Design review of the part shown in the three views and the two pictorial views. Dimensions are in mm from the part's minimum x, y and z. A direction names the side the tool comes from. Coordinates: 2 decimals unless noted, no trailing zeros. Write each loop counter-clockwise with the first axis right and the second up, starting at its lowest first coordinate (ties: lowest second). Pieces come first, ordered by that corner, then holes. Notation, with made-up numbers: (66.25, -32.5) -> (71.25, -32.5) arc R8 ccw to (71.25, -19.5) -> close; hole circle Ø11 at (13.5, 76). An arc over 180 degrees is marked (long way). Write each question's results on one line, items separated by ' | '.
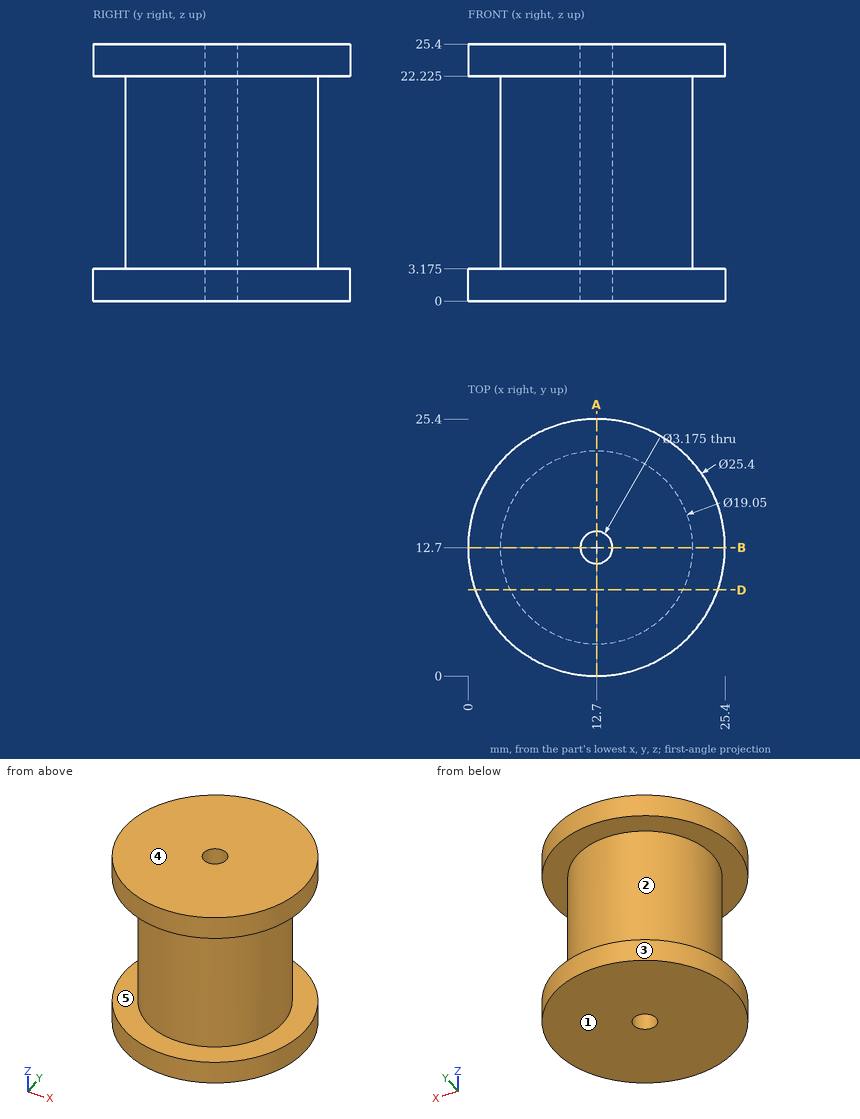
Q1. Add section D-D (y = 8.5). Write out the cut boundary in (x, z) (3 decimals), plus the area to 3 significant figures.
Solution:
outline: (0.715, 0) -> (24.685, 0) -> (24.685, 3.175) -> (21.249, 3.175) -> (21.249, 22.225) -> (24.685, 22.225) -> (24.685, 25.4) -> (0.715, 25.4) -> (0.715, 22.225) -> (4.151, 22.225) -> (4.151, 3.175) -> (0.715, 3.175) -> close | area: 478 mm²
Q2. For line 1 (Y direction, x = 12.7, z = 9.25) (1 decimal); line 2 (Y direction, x = 12.25, z = 23.5); line 3 (Z direction, x = 6.5, y = 23) (3 decimals), list the stretches that pass through material, from the lowest coordinate up. Write a range as from..to.
Solution:
line 1: 3.2..11.1, 14.3..22.2 | line 2: 0.01..11.18, 14.22..25.39 | line 3: 0..3.175, 22.225..25.4
Q3. Clearance check with flat-ended pins moving along their axes: P1, Ø1, axis at x = 15, z = 22.5, coming from the -Y side; P2, Ø4, axis at y = 5.5, z = 6, coming from the -X side; P3, Ø1.5, axis at y = 5, z = 2.5, coming from the -X side. State where each tip first meets the part, or that it passes through.
Solution:
P1: y = 0.13 | P2: x = 4.72 | P3: x = 2.07
Q4. Add section A-A (x = 12.7). Write out the cut boundary in (y, z) (1 decimal).
Solution:
outline: (0, 0) -> (11.1, 0) -> (11.1, 25.4) -> (0, 25.4) -> (0, 22.2) -> (3.2, 22.2) -> (3.2, 3.2) -> (0, 3.2) -> close; (14.3, 0) -> (25.4, 0) -> (25.4, 3.2) -> (22.2, 3.2) -> (22.2, 22.2) -> (25.4, 22.2) -> (25.4, 25.4) -> (14.3, 25.4) -> close
Q5. Draft analysis for pull direction Z (two halves, no side actions). For the marked faces 1, 2 and 3, state which applies: pulls with the +Z half, pulls with the -Z half, needs draft (parallel to the pull), parting line crosses it, or undercut.
Solution:
face 1: pulls with the -Z half | face 2: undercut | face 3: needs draft
Q6. Machinability: for the marked faces 4 and 5, which of the approach directions +Z, -Z, +X, -X, +Y, -Y give a long, thin tool a straight path to every point of the face, cutting with its end or side? Answer none if there is none.
Solution:
face 4: +Z, +X, -X, +Y, -Y | face 5: none
